The figure shows three views and two pictorial views of one solid part (mm, origin at its lowest corner). Answer the questions. A direction names the side the tool comes from. Round coordinates to 2 decimals unless told otherwise and drop trailing zeros. Order: outer loops, then holes, each group sorted by start corner. A loop starts at its lowest first (then second) coordinate and runs counter-clockwise, first axis right, second up. Notation, with made-up numbers: (46.5, 33) - (60.5, 33) arc R22 ccw to (60.5, 63) - close; hole circle Ø7 at (84.5, -17). An arc over 180 degrees is marked (long way). One line per item, written item: value. Start each with the question number.
1. Section D-D, the plane z = 32.5 is taken. Give the vertices of the cut face in (x, y), then the cut area to 3 significant figures.
2. Straight lines are drawn through the part: line 1 (Z direction, x = 44, y = 6.5); line 2 (X direction, y = 27.25, z = 4.5); line 3 (Z direction, x = 95, y = 7.25). For each, find the intervals that lie inside material, in ascending order.
3. Section A-A, the plane x = 6 is taken. Give the vertices of the cut face in (y, z), then the cut area to 3 significant figures.
4. Section C-C, the plane x = 25 is taken. Give the vertices of the cut face in (y, z).
5. Section B-B, the plane z = 44 is taken. Give the vertices of the cut face in (x, y).
6. Flat-ended cylindrical pins translate along their axes: P1, Ø15, axis at x = 77.5, y = 11.5, coming from the +Z side; P2, Ø4, axis at y = 16, z = 32, coming from the +X side. Find the tip coordinate at first contact, or state that the pin passes through.
7. For a pull along X with two mould halves and no side action, classify the marked faces 3, 4 and 5 as released by +X, released by -X, zero draft, split by the parting line, or undercut.
8. A tool of negligible diameter and unlimited length cuts with its end or side. For the marked faces 1 and 2, from which of +Z, -Z, +X, -X, +Y, -Y can it reach the whole face along a straight path? Write none if from no direction.
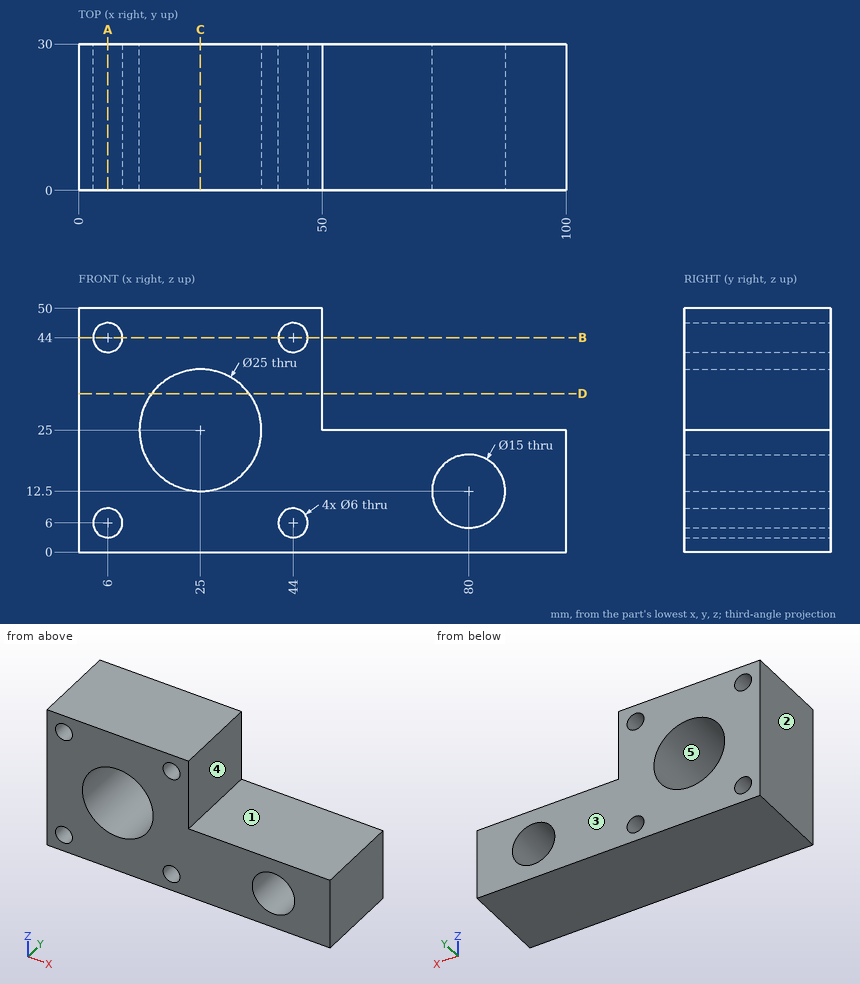
Answer list:
1. outline: (0, 0) - (15, 0) - (15, 30) - (0, 30) - close; (35, 0) - (50, 0) - (50, 30) - (35, 30) - close
1. area: 900 mm²
2. line 1: z = 0 to 3, 9 to 41, 47 to 50
2. line 2: x = 0 to 3.4, 8.6 to 41.4, 46.6 to 100
2. line 3: z = 0 to 25
3. outline: (0, 0) - (30, 0) - (30, 3) - (0, 3) - close; (0, 9) - (30, 9) - (30, 41) - (0, 41) - close; (0, 47) - (30, 47) - (30, 50) - (0, 50) - close
3. area: 1,140 mm²
4. outline: (0, 0) - (30, 0) - (30, 12.5) - (0, 12.5) - close; (0, 37.5) - (30, 37.5) - (30, 50) - (0, 50) - close
5. outline: (0, 0) - (3, 0) - (3, 30) - (0, 30) - close; (9, 0) - (41, 0) - (41, 30) - (9, 30) - close; (47, 0) - (50, 0) - (50, 30) - (47, 30) - close
6. P1: stops at z = 25
6. P2: stops at x = 50
7. face 3: zero draft
7. face 4: released by +X
7. face 5: undercut
8. face 1: +Z, +X, +Y, -Y
8. face 2: +Z, -Z, -X, +Y, -Y
